from build123d import *

# Parameters (mm, degrees)
SKETCH_1_W      = 120
SKETCH_1_H      = 120
EXTRUDE_1_DEPTH = 120
CHAMFER_1_SIZE  = 12


with BuildPart() as part:
    # 草图1 → 凸台-拉伸1 (new body)
    with BuildSketch(Plane(origin=(0, 0, 0), x_dir=(0, 0, -1), z_dir=(1, 0, 0))):
        with Locations((20.102245328, 28.139540774)):
            Rectangle(SKETCH_1_W, SKETCH_1_H)
    extrude(amount=EXTRUDE_1_DEPTH)

    # 倒角1
    chamfer_1_edges = [part.edges().sort_by_distance(p)[0] for p in [
        (120, 28.139540774, -80.102245328),
        (120, 88.139540774, -20.102245328),
        (120, 28.139540774, 39.897754672),
        (0, 88.139540774, -20.102245328),
        (0, 28.139540774, -80.102245328),
        (0, -31.860459226, -20.102245328),
        (0, 28.139540774, 39.897754672),
        (60, 88.139540774, 39.897754672),
        (60, 88.139540774, -80.102245328),
        (60, -31.860459226, -80.102245328),
        (60, -31.860459226, 39.897754672),
        (120, -31.860459226, -20.102245328),
    ]]
    chamfer(chamfer_1_edges, length=CHAMFER_1_SIZE)


solid = part.part
Can you work these out from the model? Positions are in its coordinate system, mm. Coordinates: 2 decimals unless noted, no trailing zeros. Order: outer loops, then holes, each group sorted by start corner. A loop starts at its lowest first (then second) coordinate and runs counter-clockwise, first axis right, second up. Notation, with made-up numbers: (-13.5, -19.5) - (6.5, -19.5) arc R15 ccw to (6.5, 7.5) - close; hole circle Ø5 at (57.5, -6.75). An arc over 180 degrees is marked (long way). Answer as a JSON object with one key per item and string values. Group by question number.
Q1. Imagine slicing it at B-B (z = -41). Please give me the cut outline in (x, y).
Q2. I need wall thicknesses on line 1 (X direction, y = 81, z = -35); line 2 (X direction, y = -24, z = -56.5); line 3 (Y direction, x = 10, z = -10.5). Which ranges of each line are inside material? Lowest first, please. Write a range as from..to.
Q3. Imagine slicing it at A-A (x = 98). Please give me the cut outline in (y, z).
Determined:
{
 "1": {"outline": "(0, -19.86) - (12, -31.86) - (108, -31.86) - (120, -19.86) - (120, 76.14) - (108, 88.14) - (12, 88.14) - (0, 76.14) - close"},
 "2": {"line 1": "x = 4.86..115.14", "line 2": "x = 4.14..115.86", "line 3": "y = -29.86..86.14"},
 "3": {"outline": "(-31.86, -68.1) - (-19.86, -80.1) - (76.14, -80.1) - (88.14, -68.1) - (88.14, 27.9) - (76.14, 39.9) - (-19.86, 39.9) - (-31.86, 27.9) - close"}
}
